```python
from build123d import *

# Parameters (mm, degrees)
SKETCH011_W     = 100
SKETCH011_H     = 50
PAD003_DEPTH    = 15
PAD004_DEPTH    = 100
SKETCH016_R     = 2.6
POCKET010_DEPTH = 200
PAD005_DEPTH    = 100
SKETCH027_R     = 2.6
POCKET018_DEPTH = 9
POCKET019_START = -5.75
POCKET019_DEPTH = 3.5
SKETCH029_R     = 5.5
POCKET020_DEPTH = 48
CHAMFER002_SIZE = 1.75
SKETCH031_R     = 2.6
POCKET022_DEPTH = 13
POCKET023_START = -3
POCKET023_DEPTH = 3.25


with BuildPart() as part:
    # Sketch011 (on Face1 of ShapeBinder) → Pad003 (new body)
    with BuildSketch(Plane(origin=(248, 180, 0), x_dir=(-1, 0, 0), z_dir=(0, 0, -1))):
        with Locations((124, 31)):
            Rectangle(SKETCH011_W, SKETCH011_H)
    extrude(amount=-PAD003_DEPTH)

    # Sketch012 (on Face5 of Pad003) → Pad004 (join)
    with BuildSketch(Plane(origin=(174, 180, 0), x_dir=(0, 1, 0), z_dir=(1, 0, 0))):
        Polygon((54, 15), (26.422836, 42.577164), (22.887302, 39.041631), (46.928932, 15), align=None)
        Polygon((41.272078, 15), (17.230447, 39.041631), (13.694913, 35.506097), (34.20101, 15), align=None)
    extrude(amount=-PAD004_DEPTH)

    # Sketch016 (on Face1 of Pad004) → Pocket010 (cut)
    with BuildSketch(Plane(origin=(248, 186, 0), x_dir=(1, 0, 0), z_dir=(0, -1, 0))):
        with Locations((-149, 7.5)):
            Circle(SKETCH016_R)
        with Locations((-99, 7.5)):
            Circle(SKETCH016_R)
    extrude(amount=-POCKET010_DEPTH, mode=Mode.SUBTRACT)

    # Sketch017 (on Face3 of Pocket010) → Pad005 (join)
    with BuildSketch(Plane(origin=(174, 180, 0), x_dir=(0, 1, 0), z_dir=(1, 0, 0))):
        Polygon((41.272078, 15), (44.100505, 17.828427), (46.928932, 15), align=None)
    extrude(amount=-PAD005_DEPTH)

    # Sketch027 (on Face2 of Pad005) → Pocket018 (cut)
    with BuildSketch(Plane(origin=(248, 180, 0), x_dir=(-1, 0, 0), z_dir=(0, 0, -1))):
        with Locations((116.5, 23.5)):
            Circle(SKETCH027_R)
        with Locations((131.5, 38.5)):
            Circle(SKETCH027_R)
    extrude(amount=-POCKET018_DEPTH, mode=Mode.SUBTRACT)

    # Sketch028 (on Face2 of Pocket018) → Pocket019 (cut)
    with BuildSketch(Plane(origin=(248, 180, 0), x_dir=(-1, 0, 0), z_dir=(0, 0, -1)).offset(POCKET019_START)):
        Polygon((126.775, 41.22798), (126.775, 35.77202), (131.5, 33.04404), (136.225, 35.77202), (136.225, 41.22798), (136.225, 56), (126.775, 56), align=None)
        Polygon((111.775, 26.22798), (111.775, 20.77202), (111.775, 6), (121.225, 6), (121.225, 20.77202), (121.225, 26.22798), (116.5, 28.95596), align=None)
    extrude(amount=-POCKET019_DEPTH, mode=Mode.SUBTRACT)

    # Sketch029 (on Face12 of Pocket019) → Pocket020 (cut)
    with BuildSketch(Plane(origin=(248, 236, 0), x_dir=(-1, 0, 0), z_dir=(0, 1, 0))):
        with Locations((99, 7.5)):
            Circle(SKETCH029_R)
        with Locations((149, 7.5)):
            Circle(SKETCH029_R)
    extrude(amount=-POCKET020_DEPTH, mode=Mode.SUBTRACT)

    # Chamfer002
    chamfer002_edges = [part.edges().sort_by_distance(p)[0] for p in [
        (146.4, 188, 7.5),
        (96.4, 188, 7.5),
    ]]
    chamfer(chamfer002_edges, length=CHAMFER002_SIZE)

    # Sketch031 (on Face13 of Chamfer002) → Pocket022 (cut)
    with BuildSketch(Plane(origin=(248, 236, 0), x_dir=(-1, 0, 0), z_dir=(0, 1, 0))):
        with Locations((83.75, 7.5)):
            Circle(SKETCH031_R)
        with Locations((164.25, 7.5)):
            Circle(SKETCH031_R)
    extrude(amount=-POCKET022_DEPTH, mode=Mode.SUBTRACT)

    # Sketch032 (on Face15 of Pocket022) → Pocket023 (cut)
    with BuildSketch(Plane(origin=(248, 236, 0), x_dir=(-1, 0, 0), z_dir=(0, 1, 0)).offset(POCKET023_START)):
        Polygon((81.02202, 2.775), (86.47798, 2.775), (89.20596, 7.5), (86.47798, 12.225), (81.02202, 12.225), (74, 12.225), (74, 2.775), align=None)
        Polygon((161.52202, 12.225), (158.79404, 7.5), (161.52202, 2.775), (166.97798, 2.775), (174, 2.775), (174, 12.225), (166.97798, 12.225), align=None)
    extrude(amount=-POCKET023_DEPTH, mode=Mode.SUBTRACT)


solid = part.part
```
Can you work these out from the model? Positions are in its coordinate system, mm. A direction names the side the tool comes from. Give positions to 0.01 mm unless a question says otherwise; leave off trailing zeros. Loops run counter-clockwise (first coordinate to the right, second up) from the corner with the lowest first, then second, coordinate; pieces in that order, holes last. Notation, with made-up numbers: M -21,13.25 L 30,13.25 A20 cw 30,26.25 Z; hole C -36,71.25 d4. An arc over 180 degrees is marked long. One line per item, written item: value.
(1) Suppose I cut it at A-A on x = 149. List the corners of the cut face in (y, z) for me, plus the area to 3 significant figures.
Returned:
outline: M 186,0 L 236,0 L 236,2 L 188,2 L 188,3.15 L 186.25,4.9 L 186,4.9 Z; M 186,10.1 L 186.25,10.1 L 188,11.85 L 188,13 L 236,13 L 236,15 L 234,15 L 206.42,42.58 L 202.89,39.04 L 224.1,17.83 L 221.27,15 L 197.23,39.04 L 193.69,35.51 L 214.2,15 L 186,15 Z
area: 557 mm^2
(2) Suppose I cut it at B-B on y = 226. List the corners of the cut face in (x, z) for me (3 decimals).
Returned:
outline: M 74,0 L 174,0 L 174,23 L 74,23 Z; hole C 83.75,7.5 d5.2; hole C 99,7.5 d11; hole M 111.775,5.75 L 121.225,5.75 L 121.225,9.25 L 111.775,9.25 Z; hole C 149,7.5 d11; hole C 164.25,7.5 d5.2
(3) I need wall thicknesses on line 1 (X direction, y = 204, z = 7) (3 decimals); line 2 (X direction, y = 207, z = 4); line 3 (Z direction, x = 83.75, y = 234.5). Which ranges of each line are inside material? Lowest first, please.
Returned:
line 1: 74 to 93.523, 104.477 to 126.775, 136.225 to 143.523, 154.477 to 174
line 2: 74 to 94.76, 103.24 to 144.76, 153.24 to 174
line 3: 0 to 4.9, 10.1 to 15
(4) Which directions (+Z, -Z, +X, -X, +Y, -Y) give clear straight access to the entire face, cutting with the end or side of a thin tool? Please do faces 1 (the face through (87.86, 231.4, 5.17)), 2 (the face through (129.1, 202.5, 2.8)), 3 (the face through (95, 188, 5)), 4 (the face through (124.7, 222.666, 16.394)).
Returned:
face 1: -X
face 2: -Z
face 3: +Y
face 4: +X, -X
(5) Suppose I cut it at D-D on y = 217. List the corners of the cut face in (x, z) for me (3 decimals).
Returned:
outline: M 74,0 L 114.376,0 L 114.376,5.75 L 111.775,5.75 L 111.775,9.25 L 121.225,9.25 L 121.225,5.75 L 118.624,5.75 L 118.624,0 L 174,0 L 174,19.272 L 74,19.272 Z; M 74,24.929 L 174,24.929 L 174,32 L 74,32 Z; hole C 99,7.5 d11; hole C 149,7.5 d11
(6) Will these pins go through, and if not, where does the flat tip stop? pin 1 (8 mm diameter, centred on x = 100, z = 6.5, fed in from +Y); pin 2 (6 mm diameter, centred on x = 145.5, z = 36.5, fed in from -Y); pin 3 (10.5 mm diameter, centred on x = 133.5, y = 195.5, fed in from +Z); pin 4 (4 mm diameter, centred on x = 164, z = 6.5, fed in from +Y).
Returned:
pin 1: y = 188
pin 2: y = 193.69
pin 3: z = 39.04
pin 4: y = 236
(7) We'd pull the mould along Z, two halves only. Please class faces 5 (the face through (126.775, 196, 7)), 6 (the face through (80, 233, 8)), 7 (the face through (125, 235, 15)), 8 (the face through (125, 236, 7)): released by +Z, released by -Z, zero draft, split by the parting line, or undercut.
Returned:
face 5: undercut
face 6: undercut
face 7: released by +Z
face 8: zero draft
